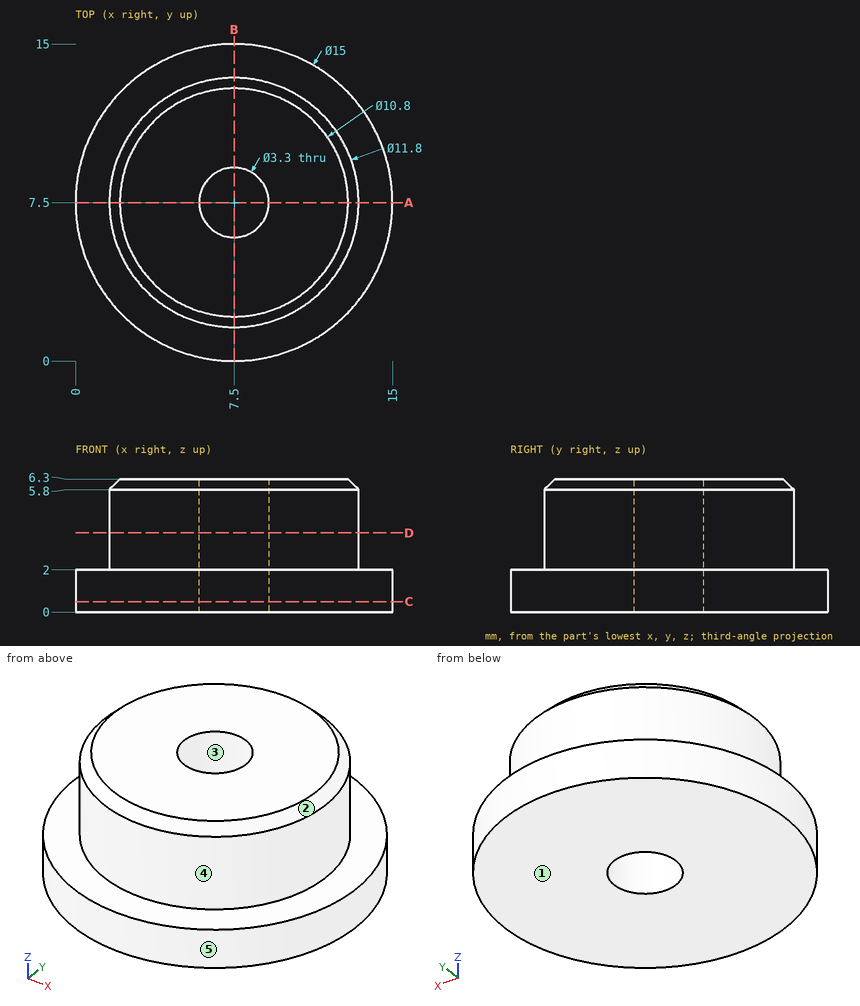
The figure shows three views and two pictorial views of one solid part (mm, origin at its lowest corner). Answer the questions. A direction names the side the tool comes from. Give positions to 0.01 mm unless a question says otherwise; leave off trailing zeros. Write each loop counter-clockwise with the first axis right and the second up, starting at its lowest first coordinate (ties: lowest second). Pieces come first, ordered by that corner, then holes. Notation, with made-up numbers: (8, 7.25) -> (22, 7.25) arc R24 ccw to (22, 41.25) -> close; hole circle Ø6 at (-12, -4.75). An arc over 180 degrees is marked (long way). Answer as a JSON object with one key per item and string values.
1) Flat-ended cylindrical pins translate along their axes: pin 1 Ø3 at (x, z) = (12.5, 5) entering from +Y; pin 2 Ø3 at (x, y) = (7.5, 7.5) entering from -Z; pin 3 Ø4 at (x, y) = (6.5, 8.5) entering from +Z; pin 4 Ø1 at (x, z) = (10, 4) entering from +Y. Find the tip coordinate at first contact, or state that the pin passes through.
Findings below:
{"pin 1": "stops at y = 12.25", "pin 2": "passes through", "pin 3": "stops at z = 6.3", "pin 4": "stops at y = 13.05"}
2) Section A-A on y = 7.5 is taken. Write down the section's boundary in (x, z), then the cut area to 3 significant figures.
Findings below:
{"outline": "(0, 0) -> (5.85, 0) -> (5.85, 6.3) -> (2.1, 6.3) -> (1.6, 5.8) -> (1.6, 2) -> (0, 2) -> close; (9.15, 0) -> (15, 0) -> (15, 2) -> (13.4, 2) -> (13.4, 5.8) -> (12.9, 6.3) -> (9.15, 6.3) -> close", "area": "59.7 mm^2"}
3) For a pull along Z with two mould halves and no side action, classify the marked faces 1, 2 and 3 as pulls with the +Z half, pulls with the -Z half, needs draft (parallel to the pull), parting line crosses it, or undercut.
Findings below:
{"face 1": "pulls with the -Z half", "face 2": "pulls with the +Z half", "face 3": "needs draft"}
4) A tool of negligible diameter and unlimited length cuts with its end or side. For the marked faces 4 and 5, from which of +Z, -Z, +X, -X, +Y, -Y can it reach the whole face along a straight path? Write none if from no direction.
Findings below:
{"face 4": "+Z", "face 5": "+Z, -Z"}
5) Straight lines are drawn through the part: probe 1 along Y at (x, z) = (7.5, 4.25); probe 2 along Z at (x, y) = (10.25, 2.25); probe 3 along Y at (x, z) = (6, 4). For each, find the intervals that lie inside material, in ascending order. Write a range as from..to.
Findings below:
{"probe 1": "y = 1.6..5.85, 9.15..13.4", "probe 2": "z = 0..2", "probe 3": "y = 1.79..6.81, 8.19..13.21"}
6) Section C-C on z = 0.5 is taken. Write down the section's boundary in (x, y), then the cut area to 3 significant figures.
Findings below:
{"outline": "circle Ø15 at (7.5, 7.5); hole circle Ø3.3 at (7.5, 7.5)", "area": "168 mm^2"}
7) Section D-D on z = 3.75 is taken. Write down the section's boundary in (x, y), then the cut area to 3 significant figures.
Findings below:
{"outline": "circle Ø11.8 at (7.5, 7.5); hole circle Ø3.3 at (7.5, 7.5)", "area": "101 mm^2"}
